```python
from build123d import *
from OCP.BRepFilletAPI import BRepFilletAPI_MakeChamfer

# Parameters (mm, degrees)
SKETCH2_R               = 67.5
SKETCH2_W               = 66.7
SKETCH2_H               = 90
BOSS_EXTRUDE1_DEPTH     = 15
SKETCH7_W               = 14
SKETCH7_H               = 11.1
CUT_EXTRUDE1_DEPTH      = 135.058839694
CUT_EXTRUDE1_DEPTH_BACK = 135.058839694
SKETCH8_R               = 9.5
FILLET1_R               = 20
SKETCH9_R               = 2.1
CUT_EXTRUDE2_DEPTH      = 97.630740606
CHAMFER1_SIZE           = 1.5
CHAMFER1_SIZE2          = 0.866025404
SKETCH10_R              = 4.1
CUT_EXTRUDE3_DEPTH      = 97.630740606
CUT_EXTRUDE4_DEPTH      = 97.630740606
SKETCH12_W              = 10
SKETCH12_H              = 5.5
BOSS_EXTRUDE2_DEPTH     = 10
BOSS_EXTRUDE3_START     = 4
SKETCH14_W              = 10
SKETCH14_H              = 3.7
BOSS_EXTRUDE3_DEPTH     = 6
BOSS_EXTRUDE4_DEPTH     = 1.3
CHAMFER2_SIZE           = 3
CHAMFER2_SIZE2          = 1.091910703
SKETCH16_W              = 10
SKETCH16_H              = 6
CUT_EXTRUDE5_DEPTH      = 97.630740606
CHAMFER3_START          = -1
CHAMFER3_DEPTH          = 16
CUT_EXTRUDE6_DEPTH      = 97.630740606


with BuildPart() as part:
    # Sketch2 → Boss-Extrude1 (new body)
    with BuildSketch(Plane(origin=(0, 0, 0), x_dir=(1, 0, 0), z_dir=(0, 1, 0))):
        with Locations(Location((0, 0, 0), (0, 0, 270))):
            Circle(SKETCH2_R)
        Rectangle(SKETCH2_W, SKETCH2_H, mode=Mode.SUBTRACT)
    extrude(amount=BOSS_EXTRUDE1_DEPTH)

    # Sketch7 → Cut-Revolve2 (revolve, cut)
    with BuildSketch(Plane(origin=(0, 15, 0), x_dir=(1, 0, 0), z_dir=(0, 1, 0))):
        with Locations((-40.35, 5.55)):
            Rectangle(SKETCH7_W, SKETCH7_H)
        with Locations((40.35, 5.55)):
            Rectangle(SKETCH7_W, SKETCH7_H)
    revolve(axis=Axis((67.5, 15, 0), (-1, 0, 0)), mode=Mode.SUBTRACT)

    # Sketch8 → Cut-Extrude1 (cut, two sides: drawn at the far end of the back side and taken through both)
    with BuildSketch(Plane.ZY.offset(-47.35).offset(-CUT_EXTRUDE1_DEPTH_BACK)):
        with Locations((0, 15)):
            Circle(SKETCH8_R)
    extrude(amount=CUT_EXTRUDE1_DEPTH + CUT_EXTRUDE1_DEPTH_BACK, mode=Mode.SUBTRACT)

    # Fillet1
    fillet1_edges = [part.edges().sort_by_distance(p)[0] for p in [
        (-33.35, 7.5, -45),
        (-33.35, 7.5, 45),
        (33.35, 7.5, 45),
        (33.35, 7.5, -45),
    ]]
    fillet(fillet1_edges, radius=FILLET1_R)

    # Sketch9 → Cut-Extrude2 (cut, through all)
    with BuildSketch(Plane(origin=(0, 15, 0), x_dir=(1, 0, 0), z_dir=(0, 1, 0))):
        with Locations(Location((-37.629775444, 17.5, 0), (0, 0, 270))):
            Circle(SKETCH9_R)
        with Locations(Location((37.629775444, 17.5, 0), (0, 0, 270))):
            Circle(SKETCH9_R)
        with Locations(Location((37.629775444, -17.5, 0), (0, 0, 270))):
            Circle(SKETCH9_R)
        with Locations(Location((-37.629775444, -17.5, 0), (0, 0, 270))):
            Circle(SKETCH9_R)
        with Locations(Location((-20, 51.23475383, 0), (0, 0, 270))):
            Circle(SKETCH9_R)
        with Locations(Location((20, 51.23475383, 0), (0, 0, 270))):
            Circle(SKETCH9_R)
        with Locations(Location((20, -51.23475383, 0), (0, 0, 270))):
            Circle(SKETCH9_R)
        with Locations(Location((-20, -51.23475383, 0), (0, 0, 270))):
            Circle(SKETCH9_R)
        with Locations(Location((0, 55, 0), (0, 0, 270))):
            Circle(SKETCH9_R)
        with Locations(Location((0, -58.5, 0), (0, 0, 270))):
            Circle(SKETCH9_R)
        with Locations(Location((46, 17.5, 0), (0, 0, 270))):
            Circle(SKETCH9_R)
        with Locations(Location((46, -17.5, 0), (0, 0, 270))):
            Circle(SKETCH9_R)
        with Locations(Location((-46, 17.5, 0), (0, 0, 270))):
            Circle(SKETCH9_R)
        with Locations(Location((-46, -17.5, 0), (0, 0, 270))):
            Circle(SKETCH9_R)
    extrude(amount=-CUT_EXTRUDE2_DEPTH, mode=Mode.SUBTRACT)

    # Chamfer1: one chamfer whose edges measure the first distance from different faces: ONE call of the kernel's chamfer builder (chamfer() names one face for all edges)
    chamfer1_edges_1 = [part.edges().sort_by_distance(p)[0] for p in [
        (-33.35, 3.9, 0),
    ]]
    chamfer1_side_1 = [part.faces().sort_by_distance(p)[0] for p in [
        (-33.35, 0.522015325, 0),
    ]]
    chamfer1_edges_2 = [part.edges().sort_by_distance(p)[0] for p in [
        (33.35, 3.9, 0),
    ]]
    chamfer1_side_2 = [part.faces().sort_by_distance(p)[0] for p in [
        (33.35, 0.522015325, 0),
    ]]
    chamfer1 = BRepFilletAPI_MakeChamfer(part.part.solid().wrapped)
    for e in chamfer1_edges_1:
        chamfer1.Add(CHAMFER1_SIZE, CHAMFER1_SIZE2, e.wrapped, chamfer1_side_1[0].wrapped)  # the first distance lies on this face
    for e in chamfer1_edges_2:
        chamfer1.Add(CHAMFER1_SIZE, CHAMFER1_SIZE2, e.wrapped, chamfer1_side_2[0].wrapped)  # the first distance lies on this face
    add(Compound.cast(chamfer1.Shape()), mode=Mode.REPLACE)

    # Sketch10 → Cut-Extrude3 (cut, through all)
    with BuildSketch(Plane.XZ):
        with Locations(Location((42.072853481, -42.072853481, 0), (0, 0, 270))):
            Circle(SKETCH10_R)
        with Locations(Location((-42.072853481, -42.072853481, 0), (0, 0, 270))):
            Circle(SKETCH10_R)
        with Locations(Location((-42.072853481, 42.072853481, 0), (0, 0, 270))):
            Circle(SKETCH10_R)
        with Locations(Location((42.072853481, 42.072853481, 0), (0, 0, 270))):
            Circle(SKETCH10_R)
    extrude(amount=-CUT_EXTRUDE3_DEPTH, mode=Mode.SUBTRACT)

    # Sketch11 → Cut-Extrude4 (cut, through all)
    with BuildSketch(Plane.XZ):
        with BuildLine():
            Line((57.5, -35.355339059), (57.5, 35.355339059))
            ThreePointArc((57.5, 35.355339059), (67.5, 0), (57.5, -35.355339059))
        make_face()
    extrude(amount=-CUT_EXTRUDE4_DEPTH, mode=Mode.SUBTRACT)

    # Sketch12 → Boss-Extrude2 (add)
    with BuildSketch(Plane(origin=(57.5, 0, 0), x_dir=(0, 0, -1), z_dir=(1, 0, 0))):
        with Locations((0, 2.75)):
            Rectangle(SKETCH12_W, SKETCH12_H)
    extrude(amount=BOSS_EXTRUDE2_DEPTH)

    # Sketch14 → Boss-Extrude3 (add)
    with BuildSketch(Plane(origin=(57.5, 0, 0), x_dir=(0, 0, -1), z_dir=(1, 0, 0)).offset(BOSS_EXTRUDE3_START)):
        with Locations((0, 7.35)):
            Rectangle(SKETCH14_W, SKETCH14_H)
    extrude(amount=BOSS_EXTRUDE3_DEPTH)

    # Sketch15 → Boss-Extrude4 (add)
    with BuildSketch(Plane(origin=(0, 9.2, 0), x_dir=(1, 0, 0), z_dir=(0, 1, 0))):
        Polygon((66.4, -2.2), (66.4, -1.6), (67.5, -1.6), (67.5, -5), (61.5, -5), (61.5, 5), (67.5, 5), (67.5, 1.6), (66.4, 1.6), (66.4, 2.2), (63.2, 2.2), (63.2, -2.2), align=None)
    extrude(amount=BOSS_EXTRUDE4_DEPTH)

    # Chamfer2
    chamfer2_edges = [part.edges().sort_by_distance(p)[0] for p in [
        (61.5, 10.5, 0),
    ]]
    chamfer2_side = [part.faces().sort_by_distance(p)[0] for p in [
        (61.5, 8, 0),
    ]]
    chamfer(chamfer2_edges, length=CHAMFER2_SIZE, length2=CHAMFER2_SIZE2, reference=chamfer2_side[0])

    # Sketch16 → Cut-Extrude5 (cut, through all)
    with BuildSketch(Plane.XZ):
        with Locations((0, 48)):
            Rectangle(SKETCH16_W, SKETCH16_H)
    extrude(amount=-CUT_EXTRUDE5_DEPTH, mode=Mode.SUBTRACT)

    # Chamfer3: read off the stored shape, not the designer's step
    # Chamfer3 outline → Chamfer3 (cut)
    with BuildSketch(Plane(origin=(0, 0, 0), x_dir=(1, 0, 0), z_dir=(0, 1, 0)).offset(CHAMFER3_START)):
        with BuildLine():
            Line((-14.45, -44.969727089), (-8.74275335, -51))
            Line((-8.74275335, -51), (-5, -51))
            Line((-5, -51), (-5, -45))
            Line((-5, -45), (-13.35, -45))
            ThreePointArc((-13.35, -45), (-13.900208244, -44.99243034), (-14.45, -44.969727089))
        make_face()
        with BuildLine():
            Line((5, -45), (5, -51))
            Line((5, -51), (8.74275335, -51))
            Line((8.74275335, -51), (14.45, -44.969727089))
            ThreePointArc((14.45, -44.969727089), (13.900208244, -44.99243034), (13.35, -45))
            Line((13.35, -45), (5, -45))
        make_face()
    extrude(amount=CHAMFER3_DEPTH, mode=Mode.SUBTRACT)

    # Sketch18 → Cut-Extrude6 (cut, through all)
    with BuildSketch(Plane.XZ):
        with BuildLine():
            Line((-57.5, 35.355339059), (-57.5, -35.355339059))
            ThreePointArc((-57.5, -35.355339059), (-67.5, 0), (-57.5, 35.355339059))
        make_face()
    extrude(amount=-CUT_EXTRUDE6_DEPTH, mode=Mode.SUBTRACT)


solid = part.part
```
Part model, mm, in its own coordinate system. A direction names the side the tool comes from. Round coordinates to 2 decimals unless told otherwise and drop trailing zeros. Loops run counter-clockwise (first coordinate to the right, second up) from the corner with the lowest first, then second, coordinate; pieces in that order, holes last. Notation, with made-up numbers: (13.5, -33.75) -> (51.5, -33.75) arc R26 ccw to (51.5, -0.75) -> close; hole circle Ø5 at (-37.75, 6). An arc over 180 degrees is marked (long way). Use one line per item in the form item = value. Start each with the question number.
Item 1: Band-saw the part on D-D (z = 58.5). List the corners of the cut face in (x, y), plus the area to 3 significant figures.
Item 2: Drill centre lines: line 1 along Z through (x, y) = (0.5, 8.5); line 2 along X through (y, z) = (2, 18); line 3 along Z through (x, y) = (41.5, 1.75). Where is each one in solid material? Low to high.
Item 3: Band-saw the part on C-C (x = -20). List the corners of the cut face in (y, z).
Item 4: Tool access for faces 5 (the flat face through (-38, 0, 1)), 6 (the cylindrical face through (-27.73, 7.6, 38.9)), 7 (the flat face through (59, 5.5, 0)): list every direction of +Z, -Z, +X, -X, +Y, -Y with a clear straight run to the whole face (end or side of a thin tool).
Item 5: Band-saw the part on B-B (z = -17.5). List the corners of the cut face in (x, y), plus the area to 4 significant figures.
Item 6: Drop flat-ended pins along their axis: pin 1 Ø3 at (x, y) = (60.5, 7) entering from +Z; pin 2 Ø8 at (x, y) = (-7.5, 12.5) entering from +Z; pin 3 Ø2 at (x, y) = (-31, 4) entering from -Z. Give the stop position or say it passes through.
Item 7: Two-plate mould, pull along Z, no slides. Class faces 1 (the cylindrical face through (0.963, 7.395, -67.493)), 2 (the flat face through (64, 4, 5)), 3 (the cylindrical face through (44.137, 7.605, 18.469)), 4 (the flat face through (62.054, 9.021, 0.07)): released by +Z, released by -Z, zero draft, split by the parting line, or undercut.
Item 8: Band-saw the part on A-A (z = -42.5). List the corners of the cut face in (x, y), plus the area to 3 significant figures.
Data:
q1.outline = (-33.67, 0) -> (-2.1, 0) -> (-2.1, 15) -> (-33.67, 15) -> close; (2.1, 0) -> (33.67, 0) -> (33.67, 15) -> (2.1, 15) -> close
q1.area = 947 mm^2
q2.line_1 = -67.5 to -57.04, -52.96 to -45, 51 to 56.46, 60.54 to 67.5
q2.line_2 = -57.5 to -48.04, -43.96 to -39.67, -35.59 to -33.35, 33.35 to 35.59, 39.67 to 43.96, 48.04 to 57.5
q2.line_3 = -53.24 to -46.13, -38.01 to 38.01, 46.13 to 53.24
q3.outline = (0, -64.47) -> (15, -64.47) -> (15, -53.33) -> (0, -53.33) -> close; (0, -49.13) -> (15, -49.13) -> (15, -43.86) -> (0, -43.86) -> close; (0, 43.86) -> (15, 43.86) -> (15, 49.13) -> (0, 49.13) -> close; (0, 53.33) -> (15, 53.33) -> (15, 64.47) -> (0, 64.47) -> close
q4.face_5 = +Z, -Z, +X, -X, -Y
q4.face_6 = +Y, -Y
q4.face_7 = +Z, -Z, +Y
q5.outline = (-57.5, 0) -> (-48.1, 0) -> (-48.1, 15) -> (-57.5, 15) -> close; (-43.9, 0) -> (-39.73, 0) -> (-39.73, 15) -> (-43.9, 15) -> close; (-35.53, 0) -> (-33.35, 0) -> (-33.35, 15) -> (-35.53, 15) -> close; (33.35, 0) -> (35.53, 0) -> (35.53, 15) -> (33.35, 15) -> close; (39.73, 0) -> (43.9, 0) -> (43.9, 15) -> (39.73, 15) -> close; (48.1, 0) -> (57.5, 0) -> (57.5, 15) -> (48.1, 15) -> close
q5.area = 472.5 mm^2
q6.pin_1 = 5
q6.pin_2 = 67.41
q6.pin_3 = -60.47
q7.face_1 = released by -Z
q7.face_2 = released by +Z
q7.face_3 = undercut
q7.face_4 = zero draft
q8.outline = (-52.44, 0) -> (-46.15, 0) -> (-46.15, 15) -> (-52.44, 15) -> close; (-38, 0) -> (-23.03, 0) -> (-23.03, 15) -> (-38, 15) -> close; (23.03, 0) -> (38, 0) -> (38, 15) -> (23.03, 15) -> close; (46.15, 0) -> (52.44, 0) -> (52.44, 15) -> (46.15, 15) -> close
q8.area = 638 mm^2
